Job drawing, mm, ordinate dimensions from the low corner. One solid piece. A direction names the side the tool comes from. Give positions to 0.01 mm unless a question says otherwise; leave off trailing zeros. Loops run counter-clockwise (first coordinate to the right, second up) from the corner with the lowest first, then second, coordinate; pieces in that order, holes last.
Item 1: Which spindle directions (+Z, -Z, +X, -X, +Y, -Y) get a long thin tool onto all of the face, cutting with end or side? Do the marked faces 1, 2 and 3. Say none if no direction does.
Item 2: Saw through at C-C on z = 11. Give the cut face in (x, y).
Item 3: Saw through at A-A on x = 4. Give the cut face in (y, z).
Item 4: Drop flat-ended pins along their axis: P1, Ø5.5, axis at x = 10.5, z = 10.5, coming from the +Y side; P2, Ø5.5, axis at x = 9.5, y = 32.5, coming from the +Z side. Give the stop position or say it passes through.
Item 5: Probe probe 1 along Y at (x, z) = (3.5, 6.5); probe 2 along Z at (x, y) = (17.25, 22). List the from-to ranges inside material, lowest first.
Item 6: Saw through at B-B on y = 22. Give the cut face in (x, z), plus the area to 3 significant figures.
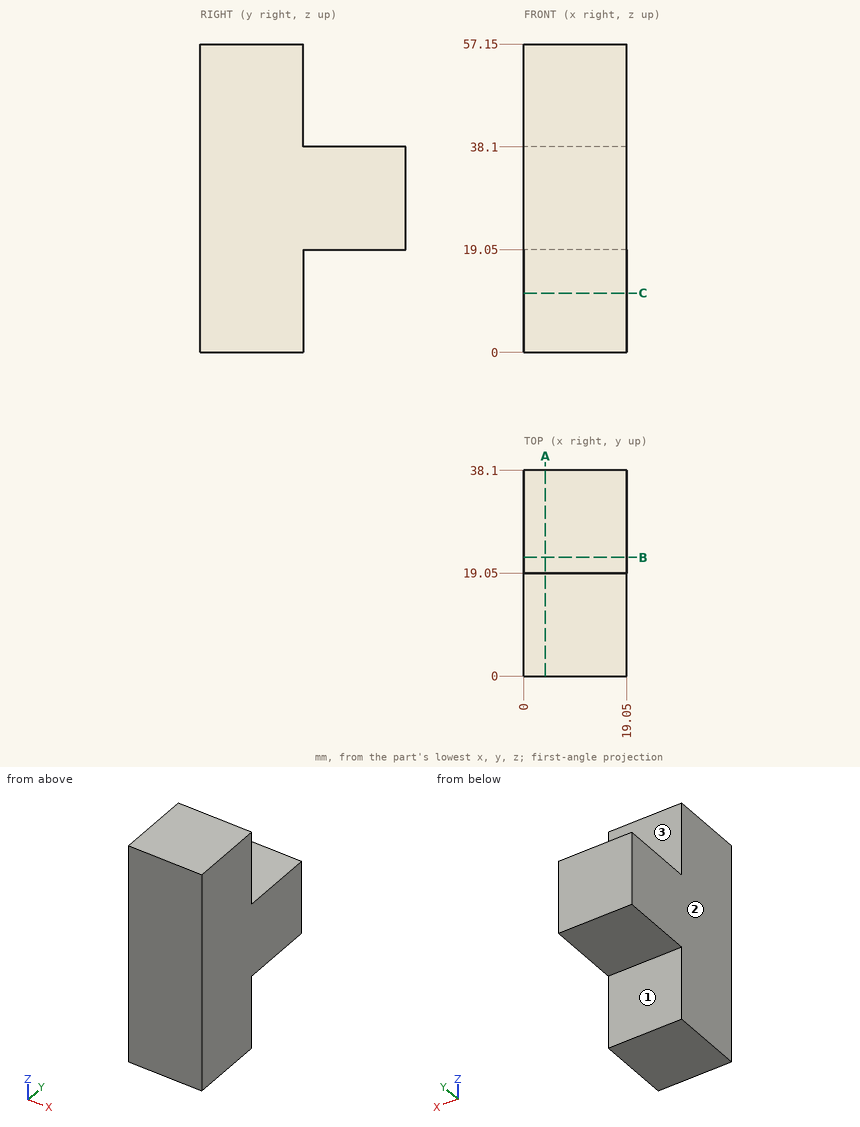
Results below:
1. face 1: -Z, +X, -X, +Y
1. face 2: +Z, -Z, -X, +Y, -Y
1. face 3: +Z, +X, -X, +Y
2. outline: (0, 0) - (19.05, 0) - (19.05, 19.05) - (0, 19.05) - close
3. outline: (0, 0) - (19.05, 0) - (19.05, 19.05) - (38.1, 19.05) - (38.1, 38.1) - (19.05, 38.1) - (19.05, 57.15) - (0, 57.15) - close
4. P1: stops at y = 19.05
4. P2: stops at z = 38.1
5. probe 1: y = 0 to 19.05
5. probe 2: z = 19.05 to 38.1
6. outline: (0, 19.05) - (19.05, 19.05) - (19.05, 38.1) - (0, 38.1) - close
6. area: 363 mm2
